```python
from build123d import *

# Parameters (mm, degrees)
F2_R     = 1.85
F3_DEPTH = 11.251
F4_R     = 4.7
F5_DEPTH = 2


with BuildPart() as f1:
    # F0 (on Right) → F1 (revolve)
    with BuildSketch(Plane.YZ):
        Polygon((11.5, 11.25), (0, 11.25), (0, 10.75), (7, 10.75), (7, 10), (10.5, 10), (10.5, 1.9), (11.5, 1.9), (11.5, 4), (19.5, 4), (19.5, 4.7), (11.5, 4.7), align=None)
    revolve(axis=Axis((0, 13.454885222, 0), (0, 1, 0)))

    # F2 (on Top) → F3 (cut, through all)
    with BuildSketch(Plane.XY):
        with Locations((0, 2.5)):
            Circle(F2_R)
    extrude(amount=F3_DEPTH, mode=Mode.SUBTRACT)

    # F4 (on face) → F5 (join)
    with BuildSketch(Plane(origin=(0, 11.5, 0), x_dir=(-1, 0, 0), z_dir=(0, 1, 0))):
        with BuildLine():
            ThreePointArc((22.627416998, -8), (23.6543654317, -4.0584474894), (24, 0))
            ThreePointArc((24, 0), (23.6543654317, 4.0584474894), (22.627416998, 8))
            Line((22.627416998, 8), (6.1119619567, 9.4449150891))
            ThreePointArc((6.1119619567, 9.4449150891), (9.88235984, 5.3760081839), (11.25, 0))
            ThreePointArc((11.25, 0), (9.88235984, -5.3760081839), (6.1119619567, -9.4449150891))
            Line((6.1119619567, -9.4449150891), (22.627416998, -8))
        make_face()
        with BuildLine():
            ThreePointArc((16.495529863, 2.9086069759), (18.3206389075, 5.5151328199), (20.9271647515, 3.6900237754))
            ThreePointArc((20.9271647515, 3.6900237754), (21.25, 0), (20.9271647515, -3.6900237754))
            ThreePointArc((20.9271647515, -3.6900237754), (18.3206389075, -5.5151328199), (16.495529863, -2.9086069759))
            ThreePointArc((16.495529863, -2.9086069759), (16.75, 0), (16.495529863, 2.9086069759))
        make_face(mode=Mode.SUBTRACT)
        with BuildLine():
            Line((-6.1119619567, 9.4449150891), (-22.627416998, 8))
            ThreePointArc((-22.627416998, 8), (-24, 0), (-22.627416998, -8))
            Line((-22.627416998, -8), (-6.1119619567, -9.4449150891))
            ThreePointArc((-6.1119619567, -9.4449150891), (-11.25, 0), (-6.1119619567, 9.4449150891))
        make_face()
        with BuildLine():
            ThreePointArc((-16.495529863, -2.9086069759), (-18.3206389075, -5.5151328199), (-20.9271647515, -3.6900237754))
            ThreePointArc((-20.9271647515, -3.6900237754), (-21.25, 0), (-20.9271647515, 3.6900237754))
            ThreePointArc((-20.9271647515, 3.6900237754), (-18.3206389075, 5.5151328199), (-16.495529863, 2.9086069759))
            ThreePointArc((-16.495529863, 2.9086069759), (-16.75, 0), (-16.495529863, -2.9086069759))
        make_face(mode=Mode.SUBTRACT)
        with BuildLine():
            ThreePointArc((11.25, 0), (9.88235984, 5.3760081839), (6.1119619567, 9.4449150891))
            ThreePointArc((6.1119619567, 9.4449150891), (0, 11.25), (-6.1119619567, 9.4449150891))
            ThreePointArc((-6.1119619567, 9.4449150891), (-11.25, 0), (-6.1119619567, -9.4449150891))
            ThreePointArc((-6.1119619567, -9.4449150891), (0, -11.25), (6.1119619567, -9.4449150891))
            ThreePointArc((6.1119619567, -9.4449150891), (9.88235984, -5.3760081839), (11.25, 0))
        make_face()
        Circle(F4_R, mode=Mode.SUBTRACT)
    extrude(amount=F5_DEPTH)


solid = f1.part
```
Can you work these out from the model? Positions are in its coordinate system, mm. A direction names the side the tool comes from. Coordinates: 2 decimals unless noted, no trailing zeros. Order: outer loops, then holes, each group sorted by start corner. A loop starts at its lowest first (then second) coordinate and runs counter-clockwise, first axis right, second up.
1. If we section it at D-D (x = -20): Please give me the cut outline in (y, z).
2. If we section it at B-B (y = 14): Please give me the cut outline in (x, z).
3. For faces 1 (the face through (21.25, 12.49, -0.05)), 2 (the face through (1.412, 16.458, 4.483)), 3 (the face through (-10, 7, 3)), which set-ups out of +Z, -Z, +X, -X, +Y, -Y let a thin tool reach every point of the face, with its end or its side?
4. If we section it at C-C (z = 8.5): Please give me the cut outline in (x, y), then the cut area to 3 significant figures.
5. I need wall thicknesses on line 1 (X direction, y = 18.75, z = 0); line 2 (X direction, y = 10.85, z = 0); line 3 (Y direction, x = -12, z = -2). Which ranges of each line are inside material? Lowest first, please.
6. If we section it at A-A (x = 0.5): Please give me the cut outline in (y, z), then the cut area to 3 significant figures.
7. Thinking about a two-plate mould opening in X: for faces 4 (the face through (24, 12, 0)), 5 (the face through (-14.49, 12.49, 8.71)), 6 (the face through (16.75, 12.49, 0.04)), which applies, +X half, -X half, draft (parallel to the pull), parting line (faces both ways), or undercut?
8. I'm going to push flat-ended pins straight in: pin 1 (1 mm diameter, centred on x = -6, y = 12, fed in from -Z); pin 2 (4 mm diameter, centred on x = -0.5, z = 0.5, fed in from +Y); pin 3 (9 mm diameter, centred on x = 0, z = 0, fed in from -Y). Where does each tip first touch, or does it pass through?
Entries:
1. outline: (11.5, -8.23) - (13.5, -8.23) - (13.5, -5.14) - (11.5, -5.14) - close; (11.5, 5.14) - (13.5, 5.14) - (13.5, 8.23) - (11.5, 8.23) - close
2. outline: circle Ø9.4 at (0, 0); hole circle Ø8 at (0, 0)
3. face 1: +Y, -Y
3. face 2: +Y
3. face 3: -Y
4. outline: (-16.91, 11.5) - (-7.37, 11.5) - (-7.37, 0) - (-6.58, 0) - (-6.58, 7) - (-5.27, 7) - (-5.27, 10.5) - (5.27, 10.5) - (5.27, 7) - (6.58, 7) - (6.58, 0) - (7.37, 0) - (7.37, 11.5) - (16.91, 11.5) - (16.91, 13.5) - (-16.91, 13.5) - close
4. area: 108 mm2
5. line 1: x = -4.7 to -4, 4 to 4.7
5. line 2: x = -11.25 to -1.9, 1.9 to 11.25
5. line 3: y = 11.5 to 13.5
6. outline: (0, -11.24) - (13.5, -11.24) - (13.5, -4.67) - (19.5, -4.67) - (19.5, -3.97) - (11.5, -3.97) - (11.5, -1.83) - (10.5, -1.83) - (10.5, -9.99) - (7, -9.99) - (7, -10.74) - (0, -10.74) - close; (0, 10.74) - (0.72, 10.74) - (0.72, 11.24) - (0, 11.24) - close; (4.28, 10.74) - (7, 10.74) - (7, 9.99) - (10.5, 9.99) - (10.5, 1.83) - (11.5, 1.83) - (11.5, 3.97) - (19.5, 3.97) - (19.5, 4.67) - (13.5, 4.67) - (13.5, 11.24) - (4.28, 11.24) - close
6. area: 70.3 mm2
7. face 4: +X half
7. face 5: -X half
7. face 6: undercut
8. pin 1: stops at z = -9.81
8. pin 2: stops at y = 11.5
8. pin 3: stops at y = 10.5
